Answer from the drawing. Dimensions are ordinates in mm from the lowest x, y and z of the part. Round coordinates to 2 decimals unless told otherwise and drop trailing zeros. Write each loop counter-clockwise with the first axis right and the second up, starting at its lowest first coordinate (ties: lowest second). Pieces come first, ordered by that corner, then holes. Notation, with made-up numbers: (20.5, 30.25) - (32.5, 30.25) arc R24 ccw to (32.5, 63.25) - close; hole circle Ø4 at (11, 50). An arc over 180 degrees is marked (long way). Answer as a JSON object with one key per item and string values.
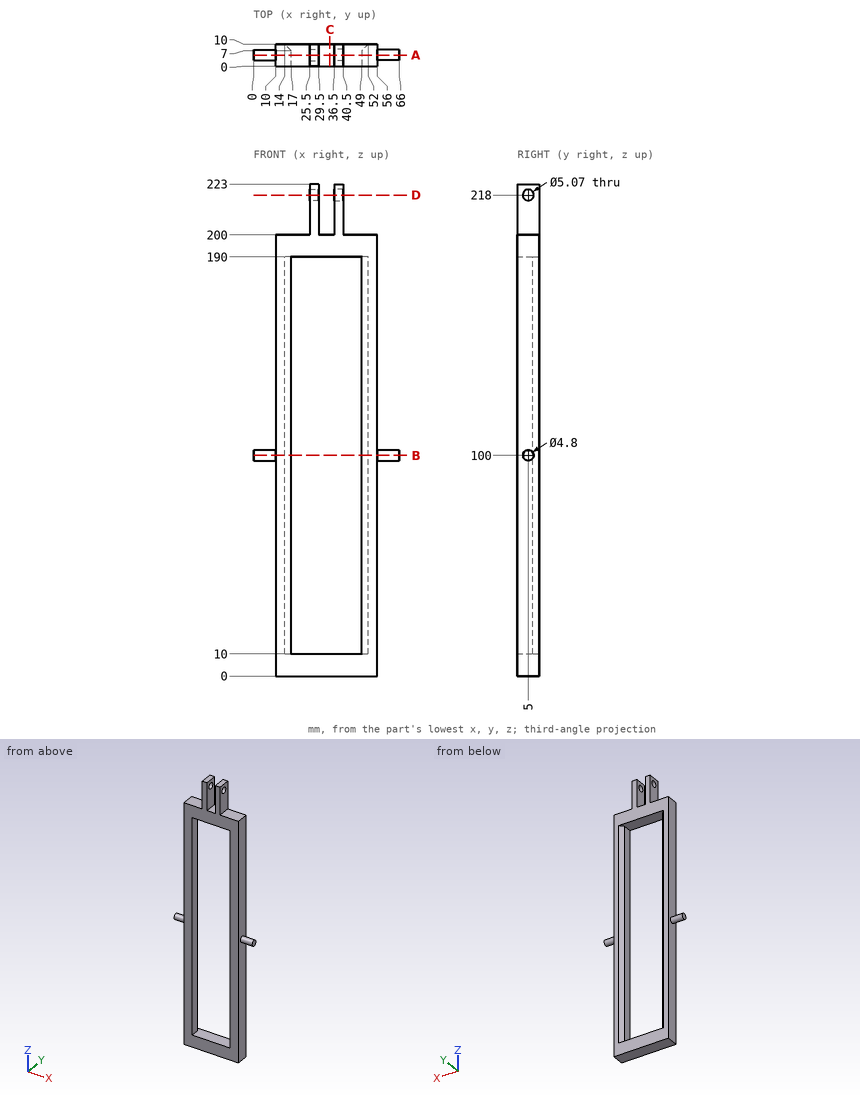
Item 1: A cutting plane is placed at C-C (x = 34.5). Write down the section's boundary in (y, z), and give its area (3 significant figures).
Results found:
{"outline": "(0, 0) - (10, 0) - (10, 10) - (0, 10) - close; (0, 190) - (10, 190) - (10, 200) - (0, 200) - close", "area": "200 mm²"}
Item 2: Each of these flat-tipped pins is pushed along its axis until it touches: P1, Ø5, axis at x = 40.5, y = 7.5, coming from the -Z side; P2, Ø3.5, axis at y = 4, z = 114.5, coming from the -X side; P3, Ø3.5, axis at y = 3, z = 79.5, coming from the +X side; P4, Ø5.5, axis at x = 33.5, y = 5.5, coming from the +Z side. Where does it stop, or does it pass through?
Results found:
{"P1": "z = 0", "P2": "x = 10", "P3": "x = 56", "P4": "z = 200"}
Item 3: A cutting plane is placed at B-B (z = 100). Write down the section's boundary in (x, y).
Results found:
{"outline": "(0, 2.6) - (10, 2.6) - (10, 0) - (17, 0) - (17, 7) - (14, 10) - (10, 10) - (10, 7.4) - (0, 7.4) - close; (49, 0) - (56, 0) - (56, 2.6) - (66, 2.6) - (66, 7.4) - (56, 7.4) - (56, 10) - (52, 10) - (49, 7) - close"}
Item 4: Consider line 1 along X through (y, z) = (3.5, 172); line 2 along Z through (x, y) = (43.5, 8.75); line 3 along Y through (x, z) = (37.45, 218) (3 decimals). Determine where each line is inside the solid, lowest interval first.
Results found:
{"line 1": "10 to 17, 49 to 56", "line 2": "0 to 10, 190 to 200", "line 3": "0 to 2.465, 7.535 to 10"}
Item 5: A cutting plane is placed at D-D (z = 218). Write down the section's boundary in (x, y) (3 decimals).
Results found:
{"outline": "(25.5, 0) - (29.5, 0) - (29.5, 2.465) - (25.5, 2.465) - close; (25.5, 7.535) - (29.5, 7.535) - (29.5, 10) - (25.5, 10) - close; (36.5, 0) - (40.5, 0) - (40.5, 2.465) - (36.5, 2.465) - close; (36.5, 7.535) - (40.5, 7.535) - (40.5, 10) - (36.5, 10) - close"}
Item 6: A cutting plane is placed at A-A (y = 5). Give the number of separate pieces and of enclosed holes in the cut face, and give its area (3 significant figures).
Results found:
{"separate pieces": "3", "enclosed holes": "1", "area": "3,680 mm²"}
